Source: three-view drawing plus pictorial views. Frame: mm from the lowest corner of the part. A direction names the side the tool comes from. Coordinates: 2 decimals unless noted, no trailing zeros. Loops run counter-clockwise (first coordinate to the right, second up) from the corner with the lowest first, then second, coordinate; pieces in that order, holes last. Notation, with made-up numbers: M -16.75,83.25 L 27.25,83.25 A38 cw 27.25,121.25 Z; hole C 17,34 d6. An arc over 180 degrees is marked long. Use a Markdown table: item, result. Add a question column.
1. Section D-D on z = 58. Output: boundary loops of the cut face in (x, y), then the cut area to 3 significant figures.
2. Set-up query: the marked faces 1, 2 and 3. Return all of +Z, -Z, +X, -X, +Y, -Y with unobstructed straight access to the full face (end or side cutting, diameter ignored); none if empty.
3. Section C-C on x = 68.5. Output: boundary loops of the cut face in (y, z), then the cut area to 3 significant figures.
4. Line query: L1, parallel to Z at x = 6, y = 73.5; L2, parallel to Y at x = 60.5, z = 35; L3, parallel to X at y = 32.5, z = 55.5. Output: solid intervals per line, ascending. Write a range as [from, to].
5. Section B-B on y = 59.5. Output: boundary loops of the cut face in (x, z), then the cut area to 3 significant figures.
6. Section A-A on z = 13. Output: boundary loops of the cut face in (x, y), then the cut area to 3 significant figures.
7. Pin query (flat end, axial travel): pin 1 (3 mm diameter, centred on y = 59, z = 48, fed in from -X); pin 2 (3 mm diameter, centred on x = 60.5, z = 51, fed in from +Y); pin 3 (1.5 mm diameter, centred on y = 71, z = 8, fed in from +X). Return the tip coordinate at first contact, or that it passes through.
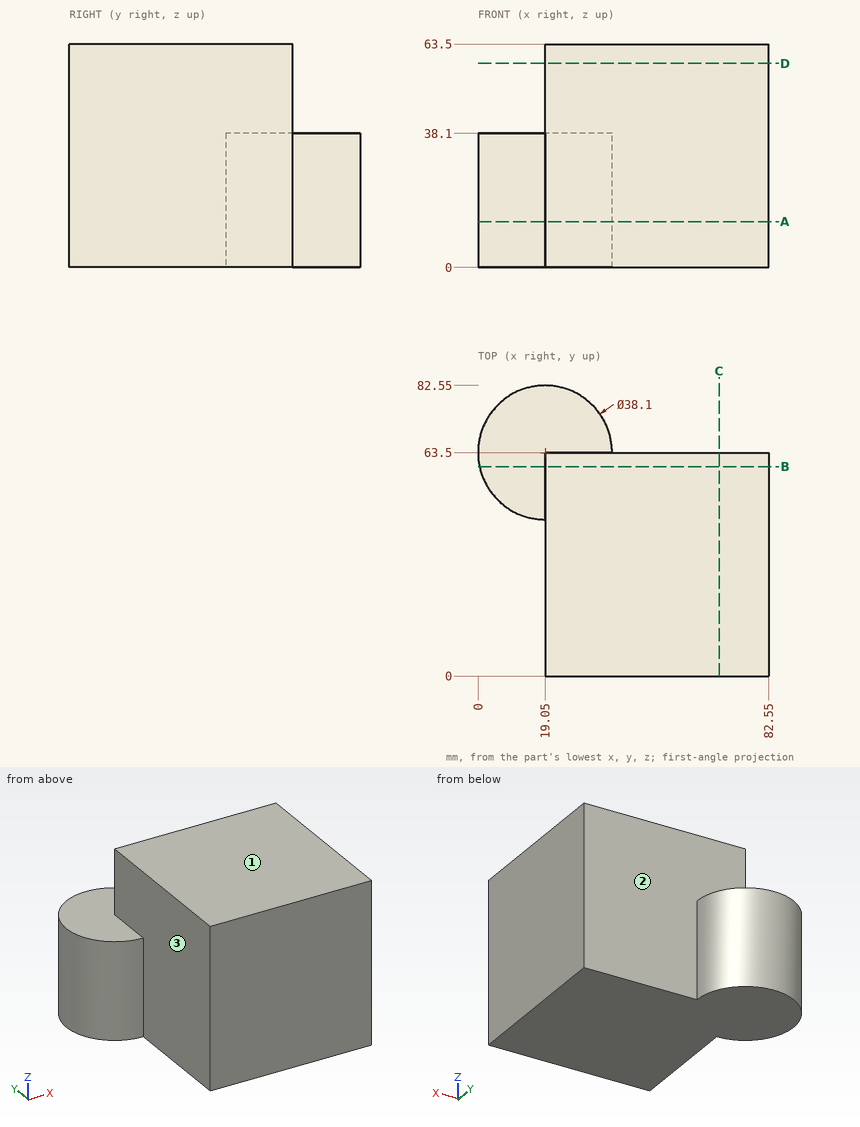
Answers below:
| question | item | result |
|---|---|---|
| 1 | outline | M 19.05,0 L 82.55,0 L 82.55,63.5 L 19.05,63.5 Z |
| 1 | area | 4,030 mm² |
| 2 | face 1 | +Z, +X, -X, +Y, -Y |
| 2 | face 2 | +Z, +X, +Y |
| 2 | face 3 | +Z, -X, -Y |
| 3 | outline | M 0,0 L 63.5,0 L 63.5,63.5 L 0,63.5 Z |
| 3 | area | 4,030 mm² |
| 4 | L1 | z = [0, 38.1] |
| 4 | L2 | y = [0, 63.5] |
| 4 | L3 | x = [19.05, 82.55] |
| 5 | outline | M 0.42,0 L 82.55,0 L 82.55,63.5 L 19.05,63.5 L 19.05,38.1 L 0.42,38.1 Z |
| 5 | area | 4,740 mm² |
| 6 | outline | M 19.05,0 L 82.55,0 L 82.55,63.5 L 38.1,63.5 A19.05 ccw long 19.05,44.45 Z |
| 6 | area | 4,890 mm² |
| 7 | pin 1 | stops at x = 19.05 |
| 7 | pin 2 | stops at y = 63.5 |
| 7 | pin 3 | stops at x = 36.86 |
